For this review, take the finished solid that the model builds, in its own axes (mm). A direction names the side the tool comes from. Coordinates: 2 decimals unless noted, no trailing zeros. Loops run counter-clockwise (first coordinate to the right, second up) from the corner with the lowest first, then second, coordinate; pieces in that order, holes last. Notation, with made-up numbers: (12, 41.25) -> (58, 41.25) arc R17 cw to (58, 72.25) -> close; hole circle Ø2 at (-16.75, 79). An arc over 180 degrees is marked (long way). One line per item, written item: value.
from build123d import *

# Parameters (mm, degrees)
SKETCH_1_W             = 100
SKETCH_1_H             = 50
SM_BASE_FLANGE_2_DEPTH = 2
OTHER_START            = -25
OTHER_1_DEPTH          = 50
OTHER_1_2_DEPTH        = 50


# Read off the part's stored shape, not the designer's step: Нарисованный сгиб1
# Sheet-metal steps are written as plain solids
with BuildPart() as part:
    # Эскиз1 → Базовая кромка2 (new body)
    with BuildSketch(Plane.XY):
        Rectangle(SKETCH_1_W, SKETCH_1_H)
    extrude(amount=-SM_BASE_FLANGE_2_DEPTH)

    # Other 1 outline → Other 1 (cut)
    with BuildSketch(Plane(origin=(0, 0, 0), x_dir=(1, 0, 0), z_dir=(0, 1, 0)).offset(OTHER_START)):
        with BuildLine():
            Line((-50, 0), (-1.271679947, 0))
            ThreePointArc((-1.271679947, 0), (-0.290344758, 1.443395312), (1.363922451, 2))
            Line((1.363922451, 2), (-50, 2))
            Line((-50, 2), (-50, 0))
        make_face()
    extrude(amount=OTHER_1_DEPTH, mode=Mode.SUBTRACT)

    # Other 1 2 outline → Other 1 2 (add)
    with BuildSketch(Plane(origin=(0, 0, 0), x_dir=(1, 0, 0), z_dir=(0, 1, 0)).offset(OTHER_START)):
        with BuildLine():
            ThreePointArc((-1.271679947, 0), (-1.347310579, -0.364854094), (-1.372677549, -0.7366))
            Line((-1.372677549, -0.7366), (-1.372677549, -49.372677549))
            Line((-1.372677549, -49.372677549), (0.627322451, -49.372677549))
            Line((0.627322451, -49.372677549), (0.627322451, -0.7366))
            ThreePointArc((0.627322451, -0.7366), (0.843067596, -0.215745145), (1.363922451, 0))
            Line((1.363922451, 0), (-1.271679947, 0))
        make_face()
    extrude(amount=OTHER_1_2_DEPTH)


solid = part.part
1. For faces 1 (the flat face through (0.627, 0, 25)), 2 (the flat face through (13, 25, -1)), list the 3-axis set-ups (+Z, -Z, +X, -X, +Y, -Y) from which the entire face can be reached by the end or side of a thin tool; tool diameter is ignored.
Return value:
face 1: +Z, +X, +Y, -Y
face 2: +Z, -Z, +X, -X, +Y
2. Take a section at C-C, the plane x = 22. Give the boundary of the cut face in (y, z).
Return value:
outline: (-25, -2) -> (25, -2) -> (25, 0) -> (-25, 0) -> close
3. Take a section at B-B, the plane z = 17.5. Give the boundary of the cut face in (x, y).
Return value:
outline: (-1.37, -25) -> (0.63, -25) -> (0.63, 25) -> (-1.37, 25) -> close
4. The part is to be moulded in two halves that separate along Z. For faces 3 (the flat face through (0, 0, 49.373)), 4 (the flat face through (-1.373, 0, 25)), 5 (the flat face through (25, 0, -2)), say which applies: pulls with the +Z half, pulls with the -Z half, needs draft (parallel to the pull), parting line crosses it, or undercut.
Return value:
face 3: pulls with the +Z half
face 4: needs draft
face 5: pulls with the -Z half
5. Take a section at A-A, the plane y = 16.5. Give the boundary of the cut face in (x, z), and give its area (3 significant figures).
Return value:
outline: (-1.37, 0.74) arc R2.74 ccw to (1.36, -2) -> (50, -2) -> (50, 0) -> (1.36, 0) arc R0.74 cw to (0.63, 0.74) -> (0.63, 49.37) -> (-1.37, 49.37) -> close
area: 200 mm2
6. Insertion check: pin 1 Ø12 at (x, y) = (20.5, 20) entering from +Z; pin 2 Ø14.5 at (y, z) = (9, 30.5) entering from +X. Each pin has a flat end and moves straight along its axis. Give the tip position at first contact, or say it passes through.
Return value:
pin 1: stops at z = 0
pin 2: stops at x = 0.63
7. To check wall thickness, follow probe 1 along X at (y, z) = (2.5, 1.5); probe 2 along Z at (x, y) = (11.5, -20); probe 3 along Z at (x, y) = (1, -10). State the ranges of each line that lie inside material, in increasing order. Write a range as from..to.
Return value:
probe 1: x = -1.37..0.63
probe 2: z = -2..0
probe 3: z = -1.98..0.1
